Work out the finished part from the listing and answer in its coordinate system (mm). Round coordinates to 2 decimals unless told otherwise and drop trailing zeros. Order: outer loops, then holes, each group sorted by start corner. A loop starts at its lowest first (then second) coordinate and runs counter-clockwise, first axis right, second up.
from build123d import *

# Parameters (mm, degrees)
SKETCH1_W                               = 224
SKETCH1_H                               = 122
BOSS_EXTRUDE1_DEPTH                     = 5
CUT_EXTRUDE1_DEPTH                      = 5
CIRPATTERN1_COUNT                       = 4
SKETCH3_R                               = 2.75
CUT_EXTRUDE5_DEPTH                      = 5
CBORE_FOR_M5_HEX_HEAD_BOLT1_D           = 5.5
CBORE_FOR_M5_HEX_HEAD_BOLT1_DEPTH       = 12.4
CBORE_FOR_M5_HEX_HEAD_BOLT1_CBORE_D     = 12.238
CBORE_FOR_M5_HEX_HEAD_BOLT1_CBORE_DEPTH = 3.5
CBORE_FOR_M5_HEX_HEAD_BOLT1_TIP         = 1.652366702
F_2_5MM_DOWEL_HOLE1_AT_2_COUNT          = 2
F_2_5MM_DOWEL_HOLE1_AT_2_PITCH          = 45
F_2_5MM_DOWEL_HOLE1_AT_3_COUNT          = 2
F_2_5MM_DOWEL_HOLE1_AT_3_PITCH          = 90
LPATTERN1_COUNT                         = 2
LPATTERN1_PITCH                         = 106.5
BOSS_EXTRUDE3_START                     = -1.5
SKETCH11_R                              = 4
SKETCH11_R_2                            = 2.75
BOSS_EXTRUDE3_DEPTH                     = 1.5
CUT_EXTRUDE6_DEPTH                      = 10
LPATTERN2_COUNT                         = 2
LPATTERN2_PITCH                         = 25
SKETCH13_R                              = 2.5
CUT_EXTRUDE7_DEPTH                      = 10
SKETCH15_W                              = 224
SKETCH15_H                              = 5
BOSS_EXTRUDE4_DEPTH                     = 18
CUT_EXTRUDE8_DEPTH                      = 5
CUT_EXTRUDE9_DEPTH                      = 10


with BuildPart() as part:
    # Sketch1 → Boss-Extrude1 (new body)
    with BuildSketch(Plane(origin=(0, 0, 0), x_dir=(1, 0, 0), z_dir=(0, 1, 0))):
        Rectangle(SKETCH1_W, SKETCH1_H)
    extrude(amount=BOSS_EXTRUDE1_DEPTH)

    # Sketch2 → Cut-Extrude1 (cut)
    with BuildSketch(Plane.XZ):
        with BuildLine():
            Line((-15, 10), (-15, -10))
            ThreePointArc((-15, -10), (-17.5, -12.5), (-20, -10))
            Line((-20, -10), (-20, 10))
            ThreePointArc((-20, 10), (-17.5, 12.5), (-15, 10))
        make_face()
    cut_extrude1 = extrude(amount=-CUT_EXTRUDE1_DEPTH, mode=Mode.SUBTRACT)

    # CirPattern1: Cut-Extrude1 ×4 about axis
    cirpattern1_axis = Axis((0, 0, 0), (0, 1, 0))
    for i in range(1, CIRPATTERN1_COUNT):
        add(cut_extrude1.rotate(cirpattern1_axis, i * 360 / CIRPATTERN1_COUNT), mode=Mode.SUBTRACT)

    # Sketch3 → Cut-Extrude5 (cut)
    with BuildSketch(Plane(origin=(0, 0, 0), x_dir=(1, 0, 0), z_dir=(0, 1, 0))):
        with Locations(Location((0, 0, 0), (0, 0, 270))):
            Circle(SKETCH3_R)
    extrude(amount=CUT_EXTRUDE5_DEPTH, mode=Mode.SUBTRACT)

    # CBORE for M5 Hex Head Bolt1
    with Locations(Plane(origin=(0, 5, 0), x_dir=(1, 0, 0), z_dir=(0, 1, 0))):
        with Locations((0, 0)):
            CounterBoreHole(CBORE_FOR_M5_HEX_HEAD_BOLT1_D / 2, CBORE_FOR_M5_HEX_HEAD_BOLT1_CBORE_D / 2, CBORE_FOR_M5_HEX_HEAD_BOLT1_CBORE_DEPTH, depth=CBORE_FOR_M5_HEX_HEAD_BOLT1_DEPTH)
            with Locations((0, 0, -(CBORE_FOR_M5_HEX_HEAD_BOLT1_DEPTH + CBORE_FOR_M5_HEX_HEAD_BOLT1_TIP / 2))):  # 118° drill point
                Cone(0, CBORE_FOR_M5_HEX_HEAD_BOLT1_D / 2, CBORE_FOR_M5_HEX_HEAD_BOLT1_TIP, mode=Mode.SUBTRACT)

    # Sketch10 → Ø2.5mm Dowel Hole1 (revolve, cut)
    with BuildSketch(Plane(origin=(109.25, 5, 45), x_dir=(0, 0, 1), z_dir=(1, 0, 0))):
        Polygon((0, 0), (0, 13.151075774), (1.25, 12.4), (1.25, 0), align=None)
    f_2_5mm_dowel_hole1 = revolve(axis=Axis((109.25, 11.35, 45), (0, -1, 0)), mode=Mode.SUBTRACT)

    # Ø2.5mm Dowel Hole1 at 2: Ø2.5mm Dowel Hole1 ×2
    with Locations(*[(0, 0, -i * F_2_5MM_DOWEL_HOLE1_AT_2_PITCH) for i in range(1, F_2_5MM_DOWEL_HOLE1_AT_2_COUNT)]):
        add(f_2_5mm_dowel_hole1, mode=Mode.SUBTRACT)

    # Ø2.5mm Dowel Hole1 at 3: Ø2.5mm Dowel Hole1 ×2
    with Locations(*[(0, 0, -i * F_2_5MM_DOWEL_HOLE1_AT_3_PITCH) for i in range(1, F_2_5MM_DOWEL_HOLE1_AT_3_COUNT)]):
        add(f_2_5mm_dowel_hole1, mode=Mode.SUBTRACT)

    # LPattern1: Ø2.5mm Dowel Hole1 ×2
    with Locations(*[(-i * LPATTERN1_PITCH, 0, 0) for i in range(1, LPATTERN1_COUNT)]):
        add(f_2_5mm_dowel_hole1, mode=Mode.SUBTRACT)

    # LPattern1 copy 1 sketch → LPattern1 copy 1 (revolve, cut)
    with BuildSketch(Plane(origin=(2.75, 5, 0), x_dir=(0, 0, 1), z_dir=(1, 0, 0))):
        Polygon((0, 0), (0, 13.151075774), (1.25, 12.4), (1.25, 0), align=None)
    revolve(axis=Axis((2.75, 11.35, 0), (0, -1, 0)), mode=Mode.SUBTRACT)

    # LPattern1 copy 2 sketch → LPattern1 copy 2 (revolve, cut)
    with BuildSketch(Plane(origin=(2.75, 5, -45), x_dir=(0, 0, 1), z_dir=(1, 0, 0))):
        Polygon((0, 0), (0, 13.151075774), (1.25, 12.4), (1.25, 0), align=None)
    revolve(axis=Axis((2.75, 11.35, -45), (0, -1, 0)), mode=Mode.SUBTRACT)

    # Sketch11 → Boss-Extrude3 (add)
    with BuildSketch(Plane(origin=(0, 1.5, 0), x_dir=(1, 0, 0), z_dir=(0, 1, 0)).offset(BOSS_EXTRUDE3_START)):
        Circle(SKETCH11_R)
        with Locations(Location((0, 0, 0), (0, 0, 270))):
            Circle(SKETCH11_R_2, mode=Mode.SUBTRACT)
    extrude(amount=BOSS_EXTRUDE3_DEPTH)

    # Sketch12 → Cut-Extrude6 (cut)
    with BuildSketch(Plane(origin=(0, 5, 0), x_dir=(1, 0, 0), z_dir=(0, 1, 0))):
        with BuildLine():
            Line((-94, -15), (-92, -15))
            ThreePointArc((-92, -15), (-89, -12), (-92, -9))
            Line((-92, -9), (-94, -9))
            ThreePointArc((-94, -9), (-97, -12), (-94, -15))
        make_face()
        with BuildLine():
            Line((-56, -15), (-54, -15))
            ThreePointArc((-54, -15), (-51, -12), (-54, -9))
            Line((-54, -9), (-56, -9))
            ThreePointArc((-56, -9), (-59, -12), (-56, -15))
        make_face()
    cut_extrude6 = extrude(amount=-CUT_EXTRUDE6_DEPTH, mode=Mode.SUBTRACT)

    # LPattern2: Cut-Extrude6 ×2
    with Locations(*[(0, 0, -i * LPATTERN2_PITCH) for i in range(1, LPATTERN2_COUNT)]):
        add(cut_extrude6, mode=Mode.SUBTRACT)

    # Sketch13 → Cut-Extrude7 (cut)
    with BuildSketch(Plane(origin=(0, 5, 0), x_dir=(1, 0, 0), z_dir=(0, 1, 0))):
        with Locations(Location((-98.5, -42.2, 0), (0, 0, 270))):
            Circle(SKETCH13_R)
        with Locations(Location((-49.5, -42.2, 0), (0, 0, 270))):
            Circle(SKETCH13_R)
    extrude(amount=-CUT_EXTRUDE7_DEPTH, mode=Mode.SUBTRACT)

    # Sketch15 → Boss-Extrude4 (add)
    with BuildSketch(Plane.XY.offset(61)):
        with Locations((0, 2.5)):
            Rectangle(SKETCH15_W, SKETCH15_H)
    extrude(amount=BOSS_EXTRUDE4_DEPTH)

    # Sketch14 → Cut-Extrude8 (cut)
    with BuildSketch(Plane(origin=(0, 5, 0), x_dir=(1, 0, 0), z_dir=(0, 1, 0))):
        with BuildLine():
            Line((29.5, -68), (27.5, -68))
            ThreePointArc((27.5, -68), (24.5, -71), (27.5, -74))
            Line((27.5, -74), (29.5, -74))
            ThreePointArc((29.5, -74), (32.5, -71), (29.5, -68))
        make_face()
    extrude(amount=-CUT_EXTRUDE8_DEPTH, mode=Mode.SUBTRACT)

    # Sketch16 → Cut-Extrude9 (cut)
    with BuildSketch(Plane(origin=(0, 5, 0), x_dir=(1, 0, 0), z_dir=(0, 1, 0))):
        with BuildLine():
            Line((-13, 10.7), (-13, -1.3))
            ThreePointArc((-13, -1.3), (-11.5, -2.8), (-10, -1.3))
            Line((-10, -1.3), (-10, 10.7))
            ThreePointArc((-10, 10.7), (-11.5, 12.2), (-13, 10.7))
        make_face()
        with BuildLine():
            Line((-25, 10.7), (-25, -1.3))
            ThreePointArc((-25, -1.3), (-23.5, -2.8), (-22, -1.3))
            Line((-22, -1.3), (-22, 10.7))
            ThreePointArc((-22, 10.7), (-23.5, 12.2), (-25, 10.7))
        make_face()
    extrude(amount=-CUT_EXTRUDE9_DEPTH, mode=Mode.SUBTRACT)


solid = part.part
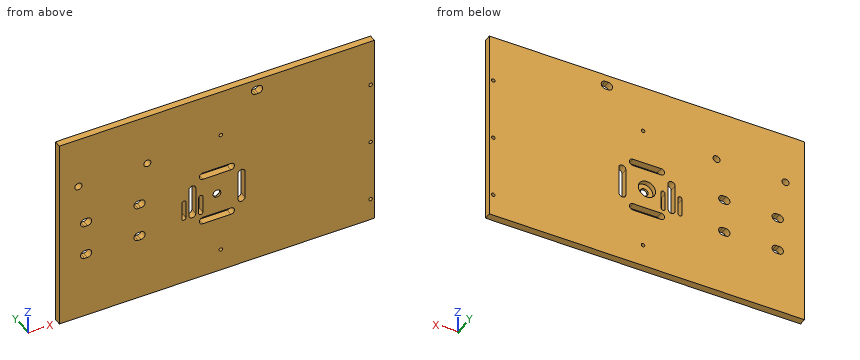
Item 1: Find section C-C (y = 3.85). State how many separate pieces and enclosed holes the cut face has, plus the area to 3 significant figures.
Item 2: Find the intervals of material crossed by line 1 along X through (y, z) = (3, -45); line 2 along X through (y, z) = (1.2, 42.2); line 3 along Z through (x, y) = (27, 2.8), in increasing order.
Item 3: Given pin 1 (2 mm diameter, centred on x = 2.75, z = 45, fed in from -Y), flat-ended and moving along its own axis, determine where the tip first touches the part or whether it passes through.
Item 4: Find section B-B (z = 17.5). Write down the section's boundary in (x, y), plus the area to 3 significant figures.
Item 5: Find section A-A (x = 17.5). Write down the section's boundary in (y, z), plus the area to 3 significant figures.
Model answer:
1. separate pieces: 1
1. enclosed holes: 19
1. area: 30,400 mm2
2. line 1: x = -112 to 1.5, 4 to 108, 110.5 to 112
2. line 2: x = -112 to -101, -96 to -52, -47 to 112
2. line 3: z = -61 to 68.04, 73.96 to 79
3. pin 1: passes through
4. outline: (-112, 0) - (-12.5, 0) - (-12.5, 5) - (-112, 5) - close; (12.5, 0) - (112, 0) - (112, 5) - (12.5, 5) - close
4. area: 995 mm2
5. outline: (0, -61) - (5, -61) - (5, -12.5) - (0, -12.5) - close; (0, 12.5) - (5, 12.5) - (5, 79) - (0, 79) - close
5. area: 575 mm2
